The model under review builds one solid part; all positions refer to its coordinate system, in mm. Round coordinates to 2 decimals unless told otherwise and drop trailing zeros. Order: outer loops, then holes, each group sorted by start corner. A loop starts at its lowest first (then second) coordinate and runs counter-clockwise, first axis right, second up. Notation, with made-up numbers: M 4,69 L 38,69 A17 cw 38,89 Z; hole C -19.5,-27.5 d11. An arc over 180 degrees is marked long. Answer as a JSON object with one key per item and string values. Group by question number.
1) Consider section A-A, the plane z = 39.5. Write out the cut boundary in (x, y), then the cut area to 3 significant figures.
2) To check wall thickness, follow line 1 (Y direction, x = 24, z = 5); line 2 (Y direction, x = 51, z = 26.5); line 3 (X direction, y = 20.5, z = 11.5). State the ranges of each line that lie inside material, in increasing order.
3) Insertion check: pin 1 Ø2 at (y, z) = (-59, 25) entering from +X; pin 2 Ø4 at (y, z) = (16, 41.5) entering from -X; pin 3 Ø12 at (y, z) = (10, 50.5) entering from +X. Each pin has a flat end and moves straight along its axis. Give the tip position at first contact, or say it passes through.
```python
from build123d import *

# Parameters (mm, degrees)
F1_DEPTH = 65.278
F2_R     = 5.08


with BuildPart() as f1:
    # F0 (on Top) → F1 (new body)
    with BuildSketch(Plane.XY):
        Polygon((33.223204, 29.108401), (-32.918401, 29.108401), (-56.692801, 0), (-56.692801, -55.016398), (-33.8328, -74.218802), (39.624002, -74.218802), (60.960002, -51.968399), (60.960002, 0), align=None)
    extrude(amount=F1_DEPTH)

    # F2
    f2_edges = [f1.edges().sort_by_distance(p)[0] for p in [
        (33.223204, 29.108401, 32.639),
        (-32.918401, 29.108401, 32.639),
        (0.152402, 29.108401, 0),
        (0.152402, 29.108401, 65.278),
        (60.960002, 0, 32.639),
        (47.091603, 14.554201, 0),
        (47.091603, 14.554201, 65.278),
        (-56.692801, 0, 32.639),
        (-44.805601, 14.554201, 0),
        (-44.805601, 14.554201, 65.278),
        (-56.692801, -55.016398, 32.639),
        (-56.692801, -27.508199, 0),
        (-56.692801, -27.508199, 65.278),
        (-33.8328, -74.218802, 32.639),
        (-45.262801, -64.6176, 0),
        (-45.262801, -64.6176, 65.278),
        (39.624002, -74.218802, 32.639),
        (2.895601, -74.218802, 0),
        (2.895601, -74.218802, 65.278),
        (60.960002, -51.968399, 32.639),
        (50.292002, -63.093601, 0),
        (50.292002, -63.093601, 65.278),
        (60.960002, -25.9842, 0),
        (60.960002, -25.9842, 65.278),
    ]]
    fillet(f2_edges, radius=F2_R)


solid = f1.part
```
Results list:
{
 "1": {"outline": "M -56.69,-52.65 A5.08 ccw -54.88,-56.54 L -35.25,-73.03 A5.08 ccw -31.98,-74.22 L 37.46,-74.22 A5.08 ccw 41.12,-72.65 L 59.55,-53.44 A5.08 ccw 60.96,-49.93 L 60.96,-2.03 A5.08 ccw 59.56,1.47 L 34.72,27.53 A5.08 ccw 31.05,29.11 L -30.51,29.11 A5.08 ccw -34.44,27.24 L -55.55,1.4 A5.08 ccw -56.69,-1.81 Z", "area": "10,900 mm^2"},
 "2": {"line 1": "-74.22 to 29.11", "line 2": "-62.36 to 10.45", "line 3": "-39.95 to 41.43"},
 "3": {"pin 1": "x = 55.18", "pin 2": "x = -45.26", "pin 3": "x = 57.15"}
}
